Geometry: final body of the model. Coordinates: model frame, mm. A direction names the side the tool comes from. Round coordinates to 2 decimals unless told otherwise and drop trailing zeros. Loops run counter-clockwise (first coordinate to the right, second up) from the corner with the lowest first, then second, coordinate; pieces in that order, holes last. Notation, with made-up numbers: M 65.25,42 L 121.25,42 A15 ccw 121.25,48 Z; hole C -27.5,4.5 d1. An arc over 180 degrees is marked long. Write each question's results on one line, items separated by ' | '.
```python
from build123d import *

# Parameters (mm, degrees)
SKETCH_R      = 30
SKETCH_R_2    = 21
PAD_DEPTH     = 10
SKETCH001_R   = 25
SKETCH001_R_2 = 21
PAD001_DEPTH  = 36
SKETCH002_R   = 25
SKETCH002_R_2 = 21
PAD002_DEPTH  = 30


with BuildPart() as part:
    # Sketch → Pad (new body)
    with BuildSketch(Plane.XY):
        Circle(SKETCH_R)
        Circle(SKETCH_R_2, mode=Mode.SUBTRACT)
    extrude(amount=PAD_DEPTH)

    # Sketch001 (on Face3 of Pad) → Pad001 (join)
    with BuildSketch(Plane(origin=(0, 0, 0), x_dir=(1, 0, 0), z_dir=(0, 0, -1))):
        Circle(SKETCH001_R)
        Circle(SKETCH001_R_2, mode=Mode.SUBTRACT)
    extrude(amount=PAD001_DEPTH)

    # Sketch002 (on Face3 of Pad001) → Pad002 (join)
    with BuildSketch(Plane.XY.offset(10)):
        Circle(SKETCH002_R)
        Circle(SKETCH002_R_2, mode=Mode.SUBTRACT)
    extrude(amount=PAD002_DEPTH)


solid = part.part
```
1. Access query for faces 4 (the face through (23.846, 7.509, 24.79)), 5 (the face through (-5.7, 20.5, 40)), 6 (the face through (23.846, -7.509, -17.748)). Directions: +Z, -Z, +X, -X, +Y, -Y. A direction counts if a zero-diameter tool reaches every point of the face in a straight line with its end or side. Return the directions, or none.
Answer key:
face 4: +Z | face 5: +Z, +X, -X, +Y, -Y | face 6: -Z
2. Ray query, probe 1 along X at (y, z) = (0, -7); probe 2 along Y at (x, z) = (0, 9). Return the intervals inside material, ascending.
Answer key:
probe 1: x = -25 to -21, 21 to 25 | probe 2: y = -30 to -21, 21 to 30
3. Draft query along Y for faces 1 (the face through (-29.97, 1.32, 4.93)), 2 (the face through (-5.7, -20.5, -36)), 3 (the face through (20.03, 6.31, 1.47)). Return one class per face: pulls with the +Y half, pulls with the -Y half, needs draft (parallel to the pull), parting line crosses it, or undercut.
Answer key:
face 1: parting line crosses it | face 2: needs draft | face 3: undercut
4. Pin query (flat end, axial travel): P1, Ø4, axis at x = 23.5, y = -16, coming from the +Z side; P2, Ø10, axis at x = 11, z = 3, coming from the +Y side; P3, Ø12, axis at y = -12, z = 30, coming from the -X side. Return the tip coordinate at first contact, or that it passes through.
Answer key:
P1: stops at z = 10 | P2: stops at y = 29.39 | P3: stops at x = -24.27
5. Section C-C (y = 23.5). Output: boundary loops of the cut face in (x, z), then the cut area to 3 significant figures.
Answer key:
outline: M -18.65,0 L -8.53,0 L -8.53,-36 L 8.53,-36 L 8.53,0 L 18.65,0 L 18.65,10 L 8.53,10 L 8.53,40 L -8.53,40 L -8.53,10 L -18.65,10 Z | area: 1,500 mm²
6. Section D-D (z = -21.5). Output: boundary loops of the cut face in (x, y).
Answer key:
outline: C 0,0 d50; hole C 0,0 d42
7. Section A-A (x = 0). Output: boundary loops of the cut face in (y, z), then the cut area to 3 significant figures.
Answer key:
outline: M -30,0 L -25,0 L -25,-36 L -21,-36 L -21,40 L -25,40 L -25,10 L -30,10 Z; M 21,-36 L 25,-36 L 25,0 L 30,0 L 30,10 L 25,10 L 25,40 L 21,40 Z | area: 708 mm²
